Geometry: final body of the model. Coordinates: model frame, mm. Give positions to 0.01 mm unless a question says otherwise; leave off trailing zeros. Write each loop counter-clockwise with the first axis right and the second up, starting at its lowest first coordinate (ties: lowest second). Pieces come first, ordered by that corner, then holes. Notation, with made-up numbers: (-12.75, 84) -> (-5.75, 84) arc R25 cw to (-5.75, 110) -> close; hole circle Ø10 at (75.25, -27). An arc over 180 degrees is marked (long way). Answer as a JSON object with one key per item and string values.
from build123d import *

# Parameters (mm, degrees)
SKETCH_1_W      = 125
SKETCH_1_H      = 165
SKETCH_1_R      = 3.1
EXTRUDE_1_DEPTH = 1
FILLET_1_R      = 10


with BuildPart() as part:
    # 草图1 → 凸台-拉伸1 (new body)
    with BuildSketch(Plane.XY):
        with Locations((55.043478261, -55.576086957)):
            Rectangle(SKETCH_1_W, SKETCH_1_H)
        with Locations((107.543478261, -128.076086957)):
            Circle(SKETCH_1_R, mode=Mode.SUBTRACT)
        with Locations((2.543478261, -128.076086957)):
            Circle(SKETCH_1_R, mode=Mode.SUBTRACT)
        with BuildLine():
            Line((107.543478261, 20.023913043), (65.043478261, 20.023913043))
            ThreePointArc((65.043478261, 20.023913043), (61.943478261, 16.923913043), (65.043478261, 13.823913043))
            Line((65.043478261, 13.823913043), (107.543478261, 13.823913043))
            ThreePointArc((107.543478261, 13.823913043), (110.643478261, 16.923913043), (107.543478261, 20.023913043))
        make_face(mode=Mode.SUBTRACT)
        with BuildLine():
            Line((45.043478261, 20.023913043), (2.543478261, 20.023913043))
            ThreePointArc((2.543478261, 20.023913043), (-0.556521739, 16.923913043), (2.543478261, 13.823913043))
            Line((2.543478261, 13.823913043), (45.043478261, 13.823913043))
            ThreePointArc((45.043478261, 13.823913043), (48.143478261, 16.923913043), (45.043478261, 20.023913043))
        make_face(mode=Mode.SUBTRACT)
    extrude(amount=EXTRUDE_1_DEPTH)

    # 圆角1
    fillet_1_edges = [part.edges().sort_by_distance(p)[0] for p in [
        (-7.456521739, 26.923913043, 0.5),
        (117.543478261, 26.923913043, 0.5),
        (117.543478261, -138.076086957, 0.5),
        (-7.456521739, -138.076086957, 0.5),
    ]]
    fillet(fillet_1_edges, radius=FILLET_1_R)


solid = part.part
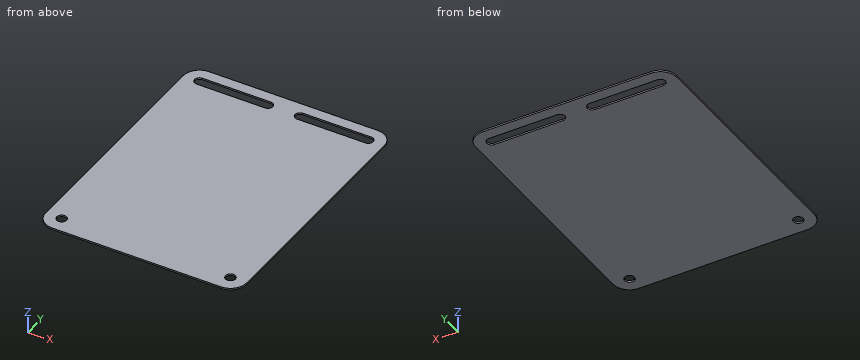
Q1. Cut plane B-B (z = 0.6). Return the cut outline in (x, y), and give its area (3 significant figures).
Values:
{"outline": "(-7.46, -128.08) arc R10 ccw to (2.54, -138.08) -> (107.54, -138.08) arc R10 ccw to (117.54, -128.08) -> (117.54, 16.92) arc R10 ccw to (107.54, 26.92) -> (2.54, 26.92) arc R10 ccw to (-7.46, 16.92) -> close; hole circle Ø6.2 at (2.54, -128.08); hole (2.54, 13.82) -> (45.04, 13.82) arc R3.1 ccw to (45.04, 20.02) -> (2.54, 20.02) arc R3.1 ccw to start; hole (65.04, 13.82) -> (107.54, 13.82) arc R3.1 ccw to (107.54, 20.02) -> (65.04, 20.02) arc R3.1 ccw to start; hole circle Ø6.2 at (107.54, -128.08)", "area": "19,900 mm²"}
Q2. Cut plane A-A (x = 79). Return the cut outline in (y, z).
Values:
{"outline": "(-138.08, 0) -> (13.82, 0) -> (13.82, 1) -> (-138.08, 1) -> close; (20.02, 0) -> (26.92, 0) -> (26.92, 1) -> (20.02, 1) -> close"}
Q3. Material intervals for L1, parallel to Y at x = 103.5, z = 0.35; L2, parallel to X at y = -130.5, z = 0.9; L3, parallel to X at y = -127.5, z = 0.6, sorted ascending. Write a range as from..to.
Values:
{"L1": "-138.08..13.82, 20.02..26.92", "L2": "-7.16..0.61, 4.48..105.61, 109.48..117.25", "L3": "-7.46..-0.5, 5.59..104.5, 110.59..117.54"}
